Design review of the part built by this model. Coordinates are the model's own, in mm. Face numbers are marked on the shaded views. A direction names the side the tool comes from. Round coordinates to 2 decimals unless told otherwise and drop trailing zeros. Loops run counter-clockwise (first coordinate to the right, second up) from the corner with the lowest first, then second, coordinate; pieces in that order, holes last. Notation, with made-up numbers: (74, 14.5) - (79, 14.5) arc R35 ccw to (79, 52.5) - close; hole circle Ø7 at (83, -18). An arc over 180 degrees is marked (long way). Use one line per item in the form item = value. Start each with the question number.
(1) Machinability: for the marked faces 1 and 2, which of the approach directions +Z, -Z, +X, -X, +Y, -Y give a long, thin tool a straight path to every point of the face, cutting with its end or side? Answer none if there is none.
(2) For pin 1 (12 mm diameter, centred on x = 32, z = 5, fed in from +Y); pin 2 (4 mm diameter, centred on y = -76.5, z = 4.5, fed in from +X); pin 3 (5 mm diameter, centred on x = 35, y = -163, fed in from +Z); pin 4 (4 mm diameter, centred on x = -19, z = 12.5, fed in from +Y), all flat-tipped, find the tip position at first contact; note any pin that passes through.
(3) We need section A-A, the plane y = -41. Write out the cut boundary in (x, z).
(4) We need section C-C, the plane z = 9.75. Give the number of separate pieces and of enclosed holes in the cut face, then the cut area to 3 significant figures.
(5) Wall thickness on probe 1 along X at (y, z) = (0, 23.3); probe 2 along X at (y, z) = (36, 24); probe 3 along Y at (x, z) = (-0.5, 13.25): over which ranges is each line inside the solid? List them lowest first. Write a range as [from, to].
(6) We need section B-B, the plane x = 19.5. Write out the cut boundary in (y, z).
(7) The part is to be moulded in two halves that separate along Y. For the marked faces 3, 4 and 5, say which applies: released by +Y, released by -Y, zero draft, split by the parting line, or undercut.
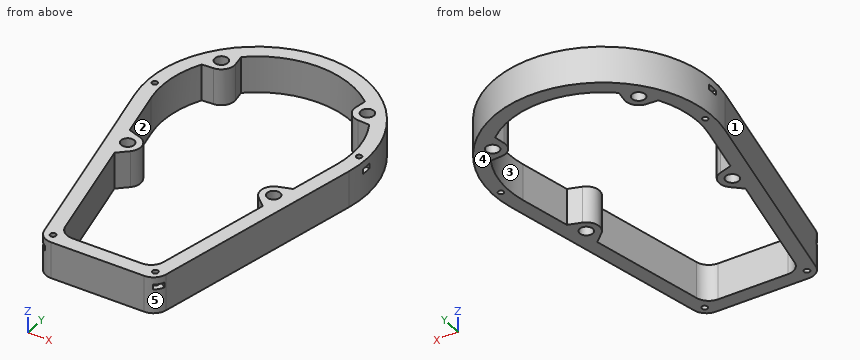
from build123d import *

# Parameters (mm, degrees)
BOSS_EXTRUDE1_DEPTH = 25
SKETCH1_R           = 1.9
SKETCH1_R_2         = 2
CUT_EXTRUDE2_DEPTH  = 188.483332593
FILLET1_R           = 10
CUT_EXTRUDE6_START  = -5
CUT_EXTRUDE6_DEPTH  = 3.4
BOSS_EXTRUDE2_DEPTH = 25
SKETCH5_R           = 4.5
CUT_EXTRUDE7_DEPTH  = 25


with BuildPart() as part:
    # Sketch2 → Boss-Extrude1 (new body)
    with BuildSketch(Plane.XY):
        with BuildLine():
            Line((-40, -170), (40, -170))
            Line((40, -170), (73.308387301, -15.839202988))
            ThreePointArc((73.308387301, -15.839202988), (0, 75), (-73.308387301, -15.839202988))
            Line((-73.308387301, -15.839202988), (-40, -170))
        make_face()
        with BuildLine():
            Line((-63.533935661, -13.727309256), (-31.929873349, -160))
            Line((-31.929873349, -160), (31.929873349, -160))
            Line((31.929873349, -160), (63.533935661, -13.727309256))
            ThreePointArc((63.533935661, -13.727309256), (0, 65), (-63.533935661, -13.727309256))
        make_face(mode=Mode.SUBTRACT)
    extrude(amount=BOSS_EXTRUDE1_DEPTH)

    # Sketch1 → Cut-Extrude2 (cut, through all)
    with BuildSketch(Plane.XY):
        with Locations((-70, 0)):
            Circle(SKETCH1_R)
        with Locations((70, 0)):
            Circle(SKETCH1_R)
        with Locations((-35, -163)):
            Circle(SKETCH1_R_2)
        with Locations((35, -163)):
            Circle(SKETCH1_R_2)
    extrude(amount=CUT_EXTRUDE2_DEPTH, mode=Mode.SUBTRACT)

    # Fillet1
    fillet1_edges = [part.edges().sort_by_distance(p)[0] for p in [
        (-31.929873349, -160, 12.5),
        (31.929873349, -160, 12.5),
        (40, -170, 12.5),
        (-40, -170, 12.5),
    ]]
    fillet(fillet1_edges, radius=FILLET1_R)

    # Sketch4 → Cut-Extrude6 (cut)
    with BuildSketch(Plane.XY.offset(25).offset(CUT_EXTRUDE6_START)):
        Polygon((-65.958548116, 0), (-67.979274058, 3.5), (-72.020725942, 3.5), (-78.181853636, 3.5), (-78.181853636, -3.5), (-72.020725942, -3.5), (-67.979274058, -3.5), align=None)
        Polygon((72.020725942, 3.5), (67.979274058, 3.5), (65.958548116, 0), (67.979274058, -3.5), (72.020725942, -3.5), (78.79506668, -3.5), (78.79506668, 3.5), align=None)
        Polygon((31.689436427, -160.681918431), (31.337200686, -164.70799137), (34.647764259, -167.02607294), (39.092604068, -170.13838328), (43.107639123, -164.40431897), (38.662799314, -161.29200863), (35.352235741, -158.97392706), align=None)
        Polygon((-34.647764259, -167.02607294), (-31.337200686, -164.70799137), (-31.689436427, -160.681918431), (-35.352235741, -158.97392706), (-38.662799314, -161.29200863), (-44.154927164, -165.137637951), (-40.139892109, -170.871702261), align=None)
    extrude(amount=-CUT_EXTRUDE6_DEPTH, mode=Mode.SUBTRACT)

    # Sketch6 → Boss-Extrude2 (add)
    with BuildSketch(Plane.XY.offset(25)):
        with BuildLine():
            Line((-50.755351044, -72.870274401), (-56.001491632, -48.589626801))
            Line((-56.001491632, -48.589626801), (-47.2213069, -51.43969249))
            ThreePointArc((-47.2213069, -51.43969249), (-41.202993524, -58.099295641), (-43.935030997, -66.649522613))
            Line((-43.935030997, -66.649522613), (-50.755351044, -72.870274401))
        make_face()
        with BuildLine():
            Line((43.935030997, -66.649522613), (50.755351044, -72.870274401))
            Line((50.755351044, -72.870274401), (56.001491632, -48.589626801))
            Line((56.001491632, -48.589626801), (47.2213069, -51.43969249))
            ThreePointArc((47.2213069, -51.43969249), (41.202993524, -58.099295641), (43.935030997, -66.649522613))
        make_face()
        with BuildLine():
            Line((-58.888367545, 30.440309427), (-42.624577683, 50.770046755))
            Line((-42.624577683, 50.770046755), (-41.11539724, 41.436604954))
            ThreePointArc((-41.11539724, 41.436604954), (-42.972180715, 34.377744572), (-49.451287154, 31.016742561))
            Line((-49.451287154, 31.016742561), (-58.888367545, 30.440309427))
        make_face()
        with BuildLine():
            Line((49.451287154, 31.016742561), (58.888367545, 30.440309427))
            Line((58.888367545, 30.440309427), (42.624577683, 50.770046755))
            Line((42.624577683, 50.770046755), (41.11539724, 41.436604954))
            ThreePointArc((41.11539724, 41.436604954), (42.972180715, 34.377744572), (49.451287154, 31.016742561))
        make_face()
    extrude(amount=-BOSS_EXTRUDE2_DEPTH)

    # Sketch5 → Cut-Extrude7 (cut)
    with BuildSketch(Plane.XY):
        with Locations((50, -60)):
            Circle(SKETCH5_R)
        with Locations((-50, -60)):
            Circle(SKETCH5_R)
        with Locations((-50, 40)):
            Circle(SKETCH5_R)
        with Locations((50, 40)):
            Circle(SKETCH5_R)
    extrude(amount=CUT_EXTRUDE7_DEPTH, mode=Mode.SUBTRACT)


solid = part.part
Data:
q1.face_1 = +Z, -Z, -X, -Y
q1.face_2 = +Z, -Z
q2.pin_1 = 70.35
q2.pin_2 = 60.63
q2.pin_3 = 25
q2.pin_4 = 73.05
q3.outline = (-67.87, 0) - (-57.64, 0) - (-57.64, 25) - (-67.87, 25) - close; (57.64, 0) - (67.87, 0) - (67.87, 25) - (57.64, 25) - close
q4.separate_pieces = 1
q4.enclosed_holes = 9
q4.area = 6,720 mm^2
q5.probe_1 = [-75, -71.9], [-68.1, -65], [65, 68.1], [71.9, 75]
q5.probe_2 = [-65.8, -52.06], [-47.94, -41.94], [41.94, 47.94], [52.06, 65.8]
q5.probe_3 = [-170, -160], [65, 75]
q6.outline = (-170, 0) - (-160, 0) - (-160, 25) - (-170, 25) - close; (62.01, 0) - (72.42, 0) - (72.42, 25) - (62.01, 25) - close
q7.face_3 = undercut
q7.face_4 = zero draft
q7.face_5 = released by -Y
